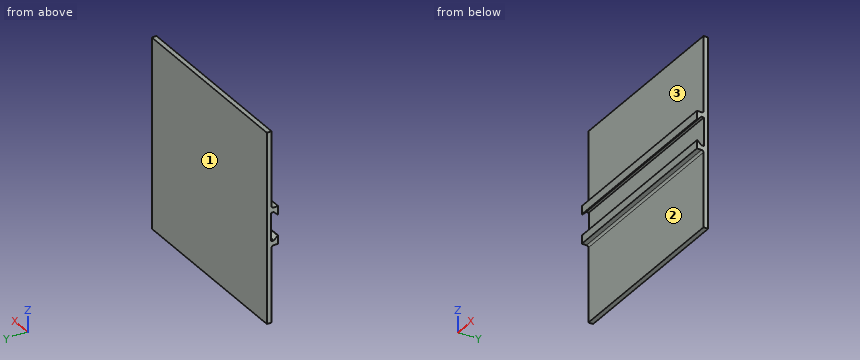
from build123d import *

# Parameters (mm, degrees)
SKETCH1_W          = 254
SKETCH1_H          = 254
BASE_DEPTH         = 6.35
SKETCH3_W          = 254
SKETCH3_H          = 50
KEY_MATERIAL_DEPTH = 8.89
KEY_SLIDE_DEPTH    = 285.119749578
KEY_CONTOURING_R   = 0.5
FILLET5_R          = 2.54


with BuildPart() as part:
    # Sketch1 → Base (new body)
    with BuildSketch(Plane(origin=(0, 0, 0), x_dir=(1, 0, 0), z_dir=(0, 1, 0))):
        Rectangle(SKETCH1_W, SKETCH1_H)
    extrude(amount=BASE_DEPTH)

    # Sketch3 → Key Material (add)
    with BuildSketch(Plane.XZ):
        Rectangle(SKETCH3_W, SKETCH3_H)
    extrude(amount=KEY_MATERIAL_DEPTH)

    # Sketch10 → Key Slide (cut, through all)
    with BuildSketch(Plane.ZY.offset(127)):
        Polygon((18.88975891, -3.047815367), (12.666574277, -9.271), (-12.649056457, -9.271), (-18.87224109, -3.047815367), (-18.87224109, 0.491), (18.88975891, 0.491), align=None)
    extrude(amount=-KEY_SLIDE_DEPTH, mode=Mode.SUBTRACT)

    # Key Contouring
    key_contouring_edges = [part.edges().sort_by_distance(p)[0] for p in [
        (0, -8.89, -13.030056457),
        (0, -8.89, 13.047574277),
        (0, -3.047815367, -18.87224109),
        (0, -3.047815367, 18.88975891),
    ]]
    fillet(key_contouring_edges, radius=KEY_CONTOURING_R)

    # Fillet5
    fillet5_edges = [part.edges().sort_by_distance(p)[0] for p in [
        (0, 0, -25),
        (0, 0, 25),
    ]]
    fillet(fillet5_edges, radius=FILLET5_R)


solid = part.part
Can you work these out from the model? Positions are in its coordinate system, mm. Face numbers are marked on the shaded views. A direction names the side the tool comes from. Give positions to 0.01 mm unless a question says otherwise; leave off trailing zeros. Loops run counter-clockwise (first coordinate to the right, second up) from the corner with the lowest first, then second, coordinate; pieces in that order, holes last. Notation, with made-up numbers: M 6,34.5 L 61,34.5 A11 cw 61,50.5 Z; hole C -24,42 d2. An arc over 180 degrees is marked long. One line per item, written item: value.
1) Please list where these lines run through material, in increasing order: line 1 (Z direction, x = -26.5, y = -2.75); line 2 (Z direction, x = -28.5, y = -7.75); line 3 (Y direction, x = -88, z = 92.5).
Geometry check:
line 1: z = -25 to -18.87, 18.89 to 25
line 2: z = -25 to -14.17, 14.19 to 25
line 3: y = 0 to 6.35
2) Imagine slicing it at A-A on x = -10.5. Write out the boundary of the cut face in (y, z).
Geometry check:
outline: M -8.89,-25 L -2.54,-25 A2.54 cw 0,-27.54 L 0,-127 L 6.35,-127 L 6.35,127 L 0,127 L 0,27.54 A2.54 cw -2.54,25 L -8.89,25 L -8.89,14.25 A0.5 ccw -8.04,13.9 L -3.19,18.74 A0.5 cw -2.84,18.89 L 0.49,18.89 L 0.49,-18.87 L -2.84,-18.87 A0.5 cw -3.19,-18.73 L -8.04,-13.88 A0.5 ccw -8.89,-14.24 Z
3) Imagine slicing it at B-B on z = 83.5. Write out the boundary of the cut face in (x, y).
Geometry check:
outline: M -127,0 L 127,0 L 127,6.35 L -127,6.35 Z
4) I'm going to push flat-ended pins straight in: pin 1 (3 mm diameter, centred on x = 25.5, y = -4.5, fed in from -Z); pin 2 (6 mm diameter, centred on x = -33, z = 92.5, fed in from -Y); pin 3 (3.5 mm diameter, centred on x = -63.5, y = -2, fed in from +Z). Where does each tip first touch, or does it pass through?
Geometry check:
pin 1: stops at z = -25
pin 2: stops at y = 0
pin 3: stops at z = 26.44
5) On a 3-axis mill with a long thin cutter (end or side, diameter ignored), from which of +Z, -Z, +X, -X, +Y, -Y can I reach the whole of each face in a straight line? I mean the marked faces 1, 2 and 3. Say none if no direction works.
Geometry check:
face 1: +Z, -Z, +X, -X, +Y
face 2: -Z, +X, -X, -Y
face 3: +Z, +X, -X, -Y
